Input: dimensioned drawing with shaded views. Units: mm. Origin: part minimum x, y, z. Coordinates: 2 decimals unless noted, no trailing zeros. Loops run counter-clockwise (first coordinate to the right, second up) from the corner with the lowest first, then second, coordinate; pieces in that order, holes last. Notation, with made-up numbers: (57.5, 2) -> (91.5, 2) arc R31 cw to (91.5, 38) -> close; hole circle Ø1 at (-28.75, -14). An arc over 180 degrees is marked (long way). Answer as CSV lines item,"result".
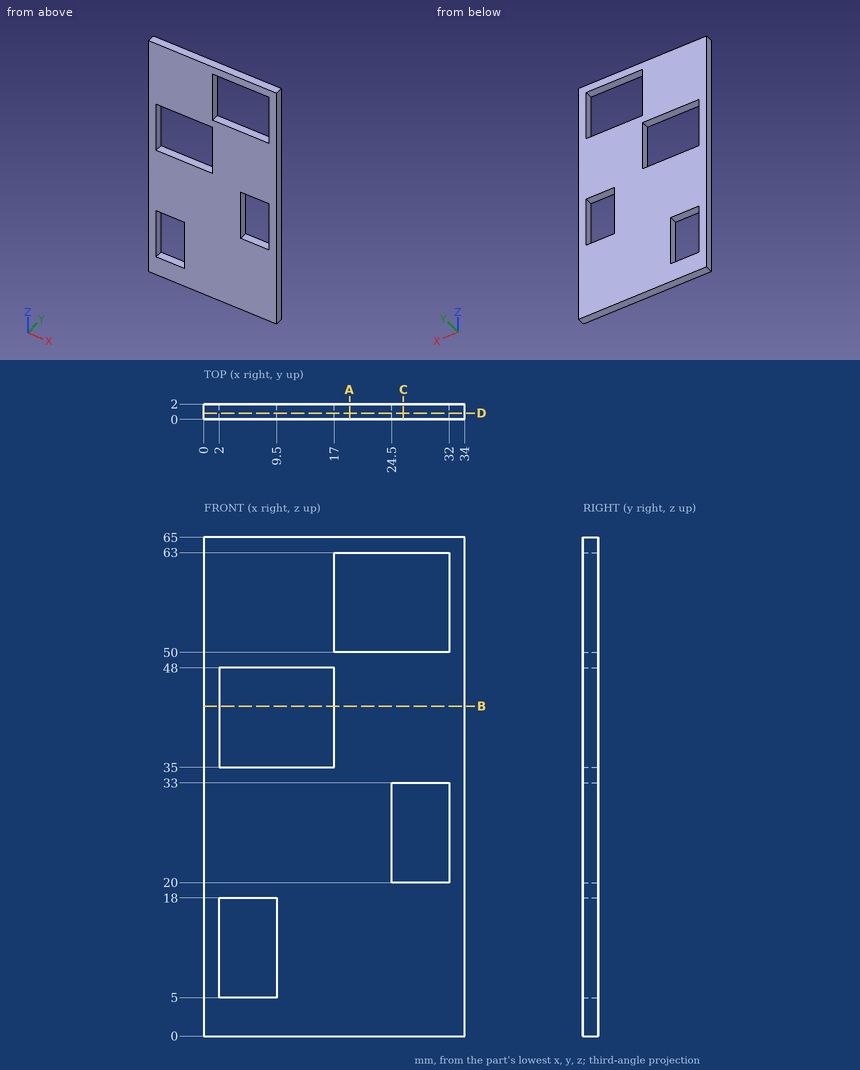
(1) Material intervals for L1, parallel to Z at x = 9, y = 0.6; L2, parallel to Z at x = 26, y = 0.3; L3, parallel to Z at x = 21, y = 1.5, sorted ascending. Write a range as [from, to].
Computed values:
L1,"[0, 5], [18, 35], [48, 65]"
L2,"[0, 20], [33, 50], [63, 65]"
L3,"[0, 50], [63, 65]"
(2) Cut plane A-A (x = 19). Return the cut outline in (y, z), then the cut area to 3 significant figures.
Computed values:
outline,"(0, 0) -> (2, 0) -> (2, 50) -> (0, 50) -> close; (0, 63) -> (2, 63) -> (2, 65) -> (0, 65) -> close"
area,"104 mm^2"
(3) Cut plane C-C (x = 26). Return the cut outline in (y, z), then the cut area to 3 significant figures.
Computed values:
outline,"(0, 0) -> (2, 0) -> (2, 20) -> (0, 20) -> close; (0, 33) -> (2, 33) -> (2, 50) -> (0, 50) -> close; (0, 63) -> (2, 63) -> (2, 65) -> (0, 65) -> close"
area,"78.0 mm^2"
(4) Cut plane D-D (y = 0.8). Return the cut outline in (x, z), then the cut area to 4 significant figures.
Computed values:
outline,"(0, 0) -> (34, 0) -> (34, 65) -> (0, 65) -> close; hole (2, 5) -> (9.5, 5) -> (9.5, 18) -> (2, 18) -> close; hole (2, 35) -> (17, 35) -> (17, 48) -> (2, 48) -> close; hole (17, 50) -> (32, 50) -> (32, 63) -> (17, 63) -> close; hole (24.5, 20) -> (32, 20) -> (32, 33) -> (24.5, 33) -> close"
area,"1,625 mm^2"
(5) Cut plane B-B (z = 43). Return the cut outline in (x, y), then the cut area to 3 significant figures.
Computed values:
outline,"(0, 0) -> (2, 0) -> (2, 2) -> (0, 2) -> close; (17, 0) -> (34, 0) -> (34, 2) -> (17, 2) -> close"
area,"38.0 mm^2"
